```python
from build123d import *

# Parameters (mm, degrees)
SKETCH1_W           = 38.1
SKETCH1_H           = 6.35
BOSS_EXTRUDE1_DEPTH = 6.35
SKETCH3_W           = 25.4
SKETCH3_H           = 6.35
BOSS_EXTRUDE2_DEPTH = 50
SKETCH6_R           = 9.35
CUT_EXTRUDE3_DEPTH  = 60.820962045
SKETCH4_R           = 2.2479
CUT_EXTRUDE1_DEPTH  = 54.600215718
SKETCH5_R           = 9.017
CUT_EXTRUDE2_DEPTH  = 60.820962045


with BuildPart() as part:
    # Sketch1 → Boss-Extrude1 (new body)
    with BuildSketch(Plane(origin=(0, 0, 0), x_dir=(1, 0, 0), z_dir=(0, 1, 0))):
        Rectangle(SKETCH1_W, SKETCH1_H)
    extrude(amount=BOSS_EXTRUDE1_DEPTH)

    # Sketch3 → Boss-Extrude2 (add)
    with BuildSketch(Plane(origin=(0, 6.35, 0), x_dir=(1, 0, 0), z_dir=(0, 1, 0))):
        Rectangle(SKETCH3_W, SKETCH3_H)
    extrude(amount=BOSS_EXTRUDE2_DEPTH)

    # Sketch6 → Cut-Extrude3 (cut, through all)
    with BuildSketch(Plane.XY.offset(3.175)):
        with Locations((0, 45)):
            Circle(SKETCH6_R)
    extrude(amount=-CUT_EXTRUDE3_DEPTH, mode=Mode.SUBTRACT)

    # Sketch4 → Cut-Extrude1 (cut, through all)
    with BuildSketch(Plane(origin=(0, 6.35, 0), x_dir=(1, 0, 0), z_dir=(0, 1, 0))):
        with Locations(Location((-15.875, 0, 0), (0, 0, 270))):
            Circle(SKETCH4_R)
        with Locations(Location((15.875, 0, 0), (0, 0, 270))):
            Circle(SKETCH4_R)
    extrude(amount=-CUT_EXTRUDE1_DEPTH, mode=Mode.SUBTRACT)

    # Sketch5 → Cut-Extrude2 (cut, through all)
    with BuildSketch(Plane.XY.offset(3.175)):
        with Locations((0, 45.25679453)):
            Circle(SKETCH5_R)
    extrude(amount=-CUT_EXTRUDE2_DEPTH, mode=Mode.SUBTRACT)


solid = part.part
```
For this review, take the finished solid that the model builds, in its own axes (mm). A direction names the side the tool comes from. Coordinates: 2 decimals unless noted, no trailing zeros. Loops run counter-clockwise (first coordinate to the right, second up) from the corner with the lowest first, then second, coordinate; pieces in that order, holes last.
1. For line 1 (X direction, y = 3.75, z = 0); line 2 (Y direction, x = 0, z = -2); line 3 (X direction, y = 28.5, z = -0.75), list the stretches that pass through material, from the lowest coordinate up.
2. Insertion check: P1, Ø1, axis at y = 30, z = -1, coming from the -X side; P2, Ø5, axis at x = -13.5, y = 38, coming from the +Z side (3 decimals). Each pin has a flat end and moves straight along its axis. Give the tip position at first contact, or say it passes through.
3. Add section B-B, the plane x = 0. Give the boundary of the cut face in (y, z) (3 decimals).
4. Add section D-D, the plane y = 30. Give the boundary of the cut face in (x, z) (3 decimals), then the cut area to 3 significant figures.
5. Add section A-A, the plane z = 0. Give the boundary of the cut face in (x, y), then the cut area to 3 significant figures.
6. Mouldability with a two-part tool opening along Z and no side actions: class faces 1 (the cylindrical face through (-2.027, 35.872, 0.044)), 2 (the cylindrical face through (13.68, 3.22, -0.49)), 3 (the flat face through (4, 22, 3.175)) as +Z half, -Z half, draft (parallel to the pull), parting line (faces both ways), or undercut.
7. Add section C-C, the plane y = 45. Give the boundary of the cut face in (x, z) (3 decimals).
8. For faces 4 (the cylindrical face through (-18.07, 3.22, -0.49)), 5 (the flat face through (-18, 6.35, -1.5)), 6 (the flat face through (14, 6.35, -2)), list the 3-axis set-ups (+Z, -Z, +X, -X, +Y, -Y) from which the entire face can be reached by the end or side of a thin tool; tool diameter is ignored.
Result:
1. line 1: x = -19.05 to -18.12, -13.63 to 13.63, 18.12 to 19.05
1. line 2: y = 0 to 35.65, 54.35 to 56.35
1. line 3: x = -12.7 to 12.7
2. P1: stops at x = -12.7
2. P2: stops at z = 3.175
3. outline: (0, -3.175) - (35.65, -3.175) - (35.65, 3.175) - (0, 3.175) - close; (54.35, -3.175) - (56.35, -3.175) - (56.35, 3.175) - (54.35, 3.175) - close
4. outline: (-12.7, -3.175) - (12.7, -3.175) - (12.7, 3.175) - (-12.7, 3.175) - close
4. area: 161 mm2
5. outline: (-19.05, 0) - (-18.12, 0) - (-18.12, 6.35) - (-19.05, 6.35) - close; (-13.63, 0) - (13.63, 0) - (13.63, 6.35) - (12.7, 6.35) - (12.7, 56.35) - (-12.7, 56.35) - (-12.7, 6.35) - (-13.63, 6.35) - close; (18.12, 0) - (19.05, 0) - (19.05, 6.35) - (18.12, 6.35) - close; hole circle Ø18.7 at (0, 45)
5. area: 1,180 mm2
6. face 1: draft
6. face 2: undercut
6. face 3: +Z half
7. outline: (-12.7, -3.175) - (-9.35, -3.175) - (-9.35, 3.175) - (-12.7, 3.175) - close; (9.35, -3.175) - (12.7, -3.175) - (12.7, 3.175) - (9.35, 3.175) - close
8. face 4: +Y, -Y
8. face 5: +Z, -Z, -X, +Y
8. face 6: +Z, -Z, +X, +Y
